Source: CAD feature listing. Evaluate the final solid. Frame: model axes, mm. A direction names the side the tool comes from. Give positions to 0.01 mm unless a question says otherwise; leave off trailing zeros. Write each loop counter-clockwise with the first axis right and the second up, starting at its lowest first coordinate (ties: lowest second). Pieces come first, ordered by that corner, then holes. Notation, with made-up numbers: (28.25, 0.25) -> (43.25, 0.25) arc R31 cw to (43.25, 26.25) -> close; hole circle Ø8 at (-15.5, -9). An arc over 180 degrees is marked (long way). Use a Markdown table: item, result. Add a question column.
```python
from build123d import *

# Parameters (mm, degrees)
SKETCH1_R           = 14.5
BOSS_EXTRUDE1_DEPTH = 2
SKETCH2_R           = 3.8
SKETCH2_R_2         = 1.5
CUT_EXTRUDE1_DEPTH  = 2.5
SKETCH3_R           = 14.5
SKETCH3_R_2         = 12.5
BOSS_EXTRUDE2_DEPTH = 23
SKETCH4_R           = 14.5
SKETCH4_R_2         = 3.8
SKETCH4_R_3         = 1.5
BOSS_EXTRUDE3_DEPTH = 1
SKETCH5_R           = 2.6
SKETCH5_R_2         = 2.5
CUT_EXTRUDE2_DEPTH  = 2
BOSS_EXTRUDE4_DEPTH = 26
SKETCH14_W          = 7
SKETCH14_H          = 26
CUT_EXTRUDE3_DEPTH  = 0.11
SKETCH16_R          = 1.5
CUT_EXTRUDE4_DEPTH  = 6
BOSS_EXTRUDE5_DEPTH = 26
SKETCH19_R          = 1.5
CUT_EXTRUDE5_DEPTH  = 5
FILLET1_R           = 5


with BuildPart() as part:
    # Sketch1 → Boss-Extrude1 (new body)
    with BuildSketch(Plane(origin=(0, 0, 0), x_dir=(1, 0, 0), z_dir=(0, 1, 0))):
        Circle(SKETCH1_R)
    extrude(amount=BOSS_EXTRUDE1_DEPTH)

    # Sketch2 → Cut-Extrude1 (cut)
    with BuildSketch(Plane(origin=(0, 2, 0), x_dir=(1, 0, 0), z_dir=(0, 1, 0))):
        Circle(SKETCH2_R)
        with Locations((-8.5, 0)):
            Circle(SKETCH2_R_2)
        with Locations((8.5, 0)):
            Circle(SKETCH2_R_2)
    extrude(amount=-CUT_EXTRUDE1_DEPTH, mode=Mode.SUBTRACT)

    # Sketch3 → Boss-Extrude2 (add)
    with BuildSketch(Plane.XZ):
        Circle(SKETCH3_R)
        Circle(SKETCH3_R_2, mode=Mode.SUBTRACT)
    extrude(amount=BOSS_EXTRUDE2_DEPTH)

    # Sketch4 → Boss-Extrude3 (add)
    with BuildSketch(Plane(origin=(0, 2, 0), x_dir=(1, 0, 0), z_dir=(0, 1, 0))):
        Circle(SKETCH4_R)
        Circle(SKETCH4_R_2, mode=Mode.SUBTRACT)
        with Locations((8.5, 0)):
            Circle(SKETCH4_R_3, mode=Mode.SUBTRACT)
        with Locations((-8.5, 0)):
            Circle(SKETCH4_R_3, mode=Mode.SUBTRACT)
    extrude(amount=BOSS_EXTRUDE3_DEPTH)

    # Sketch5 → Cut-Extrude2 (cut)
    with BuildSketch(Plane(origin=(0, 3, 0), x_dir=(1, 0, 0), z_dir=(0, 1, 0))):
        with Locations((8.5, 0)):
            Circle(SKETCH5_R)
        with Locations((-8.5, 0)):
            Circle(SKETCH5_R_2)
    extrude(amount=-CUT_EXTRUDE2_DEPTH, mode=Mode.SUBTRACT)

    # Sketch12 → Boss-Extrude4 (add)
    with BuildSketch(Plane.XZ.offset(23)):
        with BuildLine():
            Line((3.5, -25.1), (-3.5, -25.1))
            Line((-3.5, -25.1), (-3.5, -14.071247279))
            ThreePointArc((-3.5, -14.071247279), (0, -14.5), (3.5, -14.071247279))
            Line((3.5, -14.071247279), (3.5, -25.1))
        make_face()
    extrude(amount=-BOSS_EXTRUDE4_DEPTH)

    # Sketch14 → Cut-Extrude3 (cut)
    with BuildSketch(Plane(origin=(0, 0, -25.1), x_dir=(-1, 0, 0), z_dir=(0, 0, -1))):
        with Locations((0, -10)):
            Rectangle(SKETCH14_W, SKETCH14_H)
    extrude(amount=-CUT_EXTRUDE3_DEPTH, mode=Mode.SUBTRACT)

    # Sketch16 → Cut-Extrude4 (cut)
    with BuildSketch(Plane(origin=(0, 0, -24.99), x_dir=(-1, 0, 0), z_dir=(0, 0, -1))):
        with Locations((0, -2)):
            Circle(SKETCH16_R)
        with Locations((0, -12)):
            Circle(SKETCH16_R)
    extrude(amount=-CUT_EXTRUDE4_DEPTH, mode=Mode.SUBTRACT)

    # Sketch18 → Boss-Extrude5 (add, through all)
    with BuildSketch(Plane.XZ.offset(23)):
        with BuildLine():
            Line((3.5, 25.1), (-3.5, 25.1))
            Line((-3.5, 25.1), (-3.5, 14.071247279))
            ThreePointArc((-3.5, 14.071247279), (0, 14.5), (3.5, 14.071247279))
            Line((3.5, 14.071247279), (3.5, 25.1))
        make_face()
    extrude(amount=-BOSS_EXTRUDE5_DEPTH)

    # Sketch19 → Cut-Extrude5 (cut)
    with BuildSketch(Plane.XY.offset(25.1)):
        with Locations((0, -2)):
            Circle(SKETCH19_R)
        with Locations((0, -12)):
            Circle(SKETCH19_R)
    extrude(amount=-CUT_EXTRUDE5_DEPTH, mode=Mode.SUBTRACT)

    # Fillet1
    fillet1_edges = [part.edges().sort_by_distance(p)[0] for p in [
        (-3.5, -10, -14.071247279),
        (3.5, -10, -14.071247279),
        (3.5, -10, 14.071247279),
        (-3.5, -10, 14.071247279),
    ]]
    fillet(fillet1_edges, radius=FILLET1_R)


solid = part.part
```
(1) Cut plane B-B on z = 0. Return the cut outline in (x, y), then the cut area to 3 significant figures.
(2) Mould query, pull axis Y, two halves, no side actions, for faces 6 (the flat face through (3.5, -10, 21)), 7 (the flat face through (10, 1, 1)), 8 (the flat face through (0, -2, 20.1)). Classes: +Y half, -Y half, draft (parallel to the pull), parting line (faces both ways), or undercut.
(3) Cut plane C-C on y = -2. Return the cut outline in (x, z).
(4) First-contact query: pin 1 Ø6 at (x, z) = (0, 0) entering from +Y; pin 2 Ø2.5 at (x, y) = (0, -2) entering from -Z; pin 3 Ø1.5 at (y, z) = (-9, 2) entering from -X; pin 4 Ø2 at (y, z) = (-14, -19.5) entering from -X. Flat tips, straight axial feed; report the tip coordinate or a pass-through.
(5) Material intervals for L1, parallel to X at y = 0.45, z = 0; L2, parallel to Y at x = 0, z = 21.6; L3, parallel to X at y = 1.5, z = 0, sorted ascending.
(6) Cut plane D-D on z = -10. Return the cut outline in (x, y).
(7) Cut plane A-A on x = 0. Return the cut outline in (y, z), then the cut area to 3 significant figures.
(8) Access query for faces 1 (the flat face through (-3.5, -10, -21)), 2 (the flat face through (3.5, -10, -21)), 3 (the flat face through (-3.5, -10, 21)), 4 (the flat face through (3, 0, -3)), 5 (the flat face through (-7, 1, 1)). Directions: +Z, -Z, +X, -X, +Y, -Y. A direction counts if a zero-diameter tool reaches every point of the face in a straight line with its end or side. Return the directions, or none.
Output:
| question | item | result |
|---|---|---|
| 1 | outline | (-14.5, -23) -> (-12.5, -23) -> (-12.5, 0) -> (-10, 0) -> (-10, 1) -> (-11, 1) -> (-11, 3) -> (-14.5, 3) -> close; (-7, 0) -> (-3.8, 0) -> (-3.8, 3) -> (-6, 3) -> (-6, 1) -> (-7, 1) -> close; (3.8, 0) -> (7, 0) -> (7, 1) -> (5.9, 1) -> (5.9, 3) -> (3.8, 3) -> close; (10, 0) -> (12.5, 0) -> (12.5, -23) -> (14.5, -23) -> (14.5, 3) -> (11.1, 3) -> (11.1, 1) -> (10, 1) -> close |
| 1 | area | 130 mm^2 |
| 2 | face 6 | draft |
| 2 | face 7 | +Y half |
| 2 | face 8 | undercut |
| 3 | outline | (-6.32, -13.05) arc R5 cw to (-3.5, -17.55) -> (-3.5, -24.99) -> (-1.5, -24.99) -> (-1.5, -18.99) -> (1.5, -18.99) -> (1.5, -24.99) -> (3.5, -24.99) -> (3.5, -17.55) arc R5 cw to (6.32, -13.05) arc R14.5 ccw to (6.32, 13.05) arc R5 cw to (3.5, 17.55) -> (3.5, 25.1) -> (1.5, 25.1) -> (1.5, 20.1) -> (-1.5, 20.1) -> (-1.5, 25.1) -> (-3.5, 25.1) -> (-3.5, 17.55) arc R5 cw to (-6.32, 13.05) arc R14.5 ccw to start; hole circle Ø25 at (0, 0) |
| 4 | pin 1 | through |
| 4 | pin 2 | z = -18.99 |
| 4 | pin 3 | x = -14.45 |
| 4 | pin 4 | x = -3.5 |
| 5 | L1 | -14.5 to -10, -7 to -3.8, 3.8 to 7, 10 to 14.5 |
| 5 | L2 | -23 to -13.5, -10.5 to -3.5, -0.5 to 3 |
| 5 | L3 | -14.5 to -11, -6 to -3.8, 3.8 to 5.9, 11.1 to 14.5 |
| 6 | outline | (-10.5, -23) -> (-7.5, -23) -> (-7.5, 0) -> (7.5, 0) -> (7.5, -23) -> (10.5, -23) -> (10.5, 3) -> (-10.5, 3) -> close |
| 7 | outline | (-23, -24.99) -> (-13.5, -24.99) -> (-13.5, -18.99) -> (-10.5, -18.99) -> (-10.5, -24.99) -> (-3.5, -24.99) -> (-3.5, -18.99) -> (-0.5, -18.99) -> (-0.5, -24.99) -> (3, -24.99) -> (3, -3.8) -> (0, -3.8) -> (0, -12.5) -> (-23, -12.5) -> close; (-23, 12.5) -> (0, 12.5) -> (0, 3.8) -> (3, 3.8) -> (3, 25.1) -> (-0.5, 25.1) -> (-0.5, 20.1) -> (-3.5, 20.1) -> (-3.5, 25.1) -> (-10.5, 25.1) -> (-10.5, 20.1) -> (-13.5, 20.1) -> (-13.5, 25.1) -> (-23, 25.1) -> close |
| 7 | area | 639 mm^2 |
| 8 | face 1 | -Z, -X, +Y, -Y |
| 8 | face 2 | -Z, +X, +Y, -Y |
| 8 | face 3 | +Z, -X, +Y, -Y |
| 8 | face 4 | -Y |
| 8 | face 5 | +Y |
